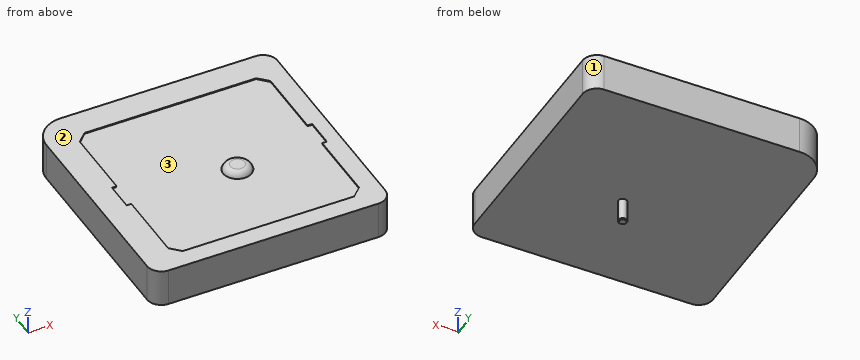
Autodesk Inventor part; units mm, degrees
ref_plane "Work Plane1" through (1.75, -1.75, 0) normal (1, 0, 0) x (0, 1, 0)
ref_plane "XZ Plane" through (0, 0, 0) normal (0, 1, 0) x (-1, 0, 0)
ref_plane "XY Plane" through (0, 0, 0) normal (0, 0, 1) x (1, 0, 0)
sketch "Sketch1" plane through (0, 0, 0) normal (0, 0, 1) x (1, 0, 0)
  line L0 (-11.05, -12.55) -> (11.05, -12.55)
  line L1 (12.55, -11.05) -> (12.55, 11.05)
  line L2 (11.05, 12.55) -> (-9.55, 12.55)
  line L3 (-12.55, 9.55) -> (-12.55, -11.05)
  line L4 (-12.55, -12.55) -> (12.55, 12.55) construction
  line L5 (12.55, -12.55) -> (-12.55, 12.55) construction
  arc A0 (-9.55, 12.55) -> (-12.55, 9.55) centre (-9.55, 9.55) ccw
  arc A1 (-12.55, -11.05) -> (-11.05, -12.55) centre (-11.05, -11.05) ccw
  arc A2 (11.05, -12.55) -> (12.55, -11.05) centre (11.05, -11.05) ccw
  arc A3 (12.55, 11.05) -> (11.05, 12.55) centre (11.05, 11.05) ccw
  circle A4 centre (1.75, -1.75) radius 0.45
  point P0 (0, 0)
  point P1 (0, 0)
  dimension "d0" = 25.1
  dimension "d1" = 3
  dimension "d2" = 0.9
  dimension "d7" = 1.5
  dimension "d8" = 25.1
  dimension "d9" = 1.75
extrude "Extrusion1" add sketch "Sketch1" along normal mid plane 4 contours A1 L3 A0 L2 A3 L1 A2 L0 | A4
extrude "Extrusion2" add sketch "Sketch1" against normal blind 4.4 and the other way blind 2.25 contours A4
chamfer "Chamfer1" distance 0.1 angle 45 1 edges at (1.3, -1.75, -4.4)
sketch "Sketch4" plane through (0, 0, 2) normal (0, 0, 1) x (1, 0, 0)
  line L0 (-12.55, 9.55) -> (-12.55, -11.05)
  arc A0 (-12.55, -11.05) -> (-11.05, -12.55) centre (-11.05, -11.05) ccw
  line L1 (-11.05, -12.55) -> (11.05, -12.55)
  arc A1 (11.05, -12.55) -> (12.55, -11.05) centre (11.05, -11.05) ccw
  line L2 (12.55, -11.05) -> (12.55, 11.05)
  arc A2 (12.55, 11.05) -> (11.05, 12.55) centre (11.05, 11.05) ccw
  line L3 (11.05, 12.55) -> (-9.55, 12.55)
  arc A3 (-9.55, 12.55) -> (-12.55, 9.55) centre (-9.55, 9.55) ccw
  line L4 (-8.55, 9.55) -> (9.55, 9.55)
  line L5 (10.55, 8.55) -> (10.55, -9.55)
  line L6 (9.55, -10.55) -> (-8.55, -10.55)
  line L7 (-9.55, -9.55) -> (-9.55, 8.55)
  line L8 (-8.55, 9.55) -> (-9.55, 8.55)
  line L9 (9.55, 9.55) -> (10.55, 8.55)
  line L10 (10.55, -9.55) -> (9.55, -10.55)
  line L11 (-8.55, -10.55) -> (-9.55, -9.55)
  line L12 (-9.55, 1) -> (-10.05, 1)
  line L13 (-10.05, 1) -> (-10.05, -2)
  line L14 (-10.05, -2) -> (-9.55, -2)
  line L15 (-9.55, -2) -> (-9.55, 1)
  line L16 (10.55, 1) -> (11.05, 1)
  line L17 (11.05, 1) -> (11.05, -2)
  line L18 (11.05, -2) -> (10.55, -2)
  line L19 (10.55, -2) -> (10.55, 1)
  point P0 (0, 0)
  point P1 (10.55, -10.55)
  point P2 (10.55, 9.55)
  point P3 (-9.55, -10.55)
  point P4 (10.55, -0.5)
  point P5 (-9.55, -0.5)
  dimension "d21" = 1
  dimension "d22" = 1
  dimension "d23" = 1
  dimension "d24" = 1
  dimension "d25" = 1
  dimension "d26" = 1
  dimension "d27" = 1
  dimension "d28" = 1
  dimension "d29" = 2
  dimension "d30" = 2
  dimension "d31" = 3
  dimension "d32" = 3
  dimension "d33" = 0.5
  dimension "d34" = 3
extrude "Extrusion3" cut sketch "Sketch4" against normal blind 0.1 contours L4 L9 L5 L10 L6 L11 L7 L8 | L7 L14 L13 L12 | L16 L17 L18 L5
ref_plane "Work Plane1" through (1.75, -1.75, 0) normal (1, 0, 0) x (0, 1, 0)
sketch "Sketch5" plane through (1.75, -1.75, 0) normal (1, 0, 0) x (0, 1, 0)
  line L0 (10.3, 1.9) -> (2.75, 1.9)
  line L1 (11.3, 1.9) -> (10.3, 1.9)
  line L2 (10.3, 1.9) -> (11.3, 1.9)
  line L3 (2.75, 1.9) -> (10.3, 1.9)
  line L4 (-0.25, 1.9) -> (2.75, 1.9)
  line L5 (-7.8, 1.9) -> (-0.25, 1.9)
  line L6 (-8.8, 1.9) -> (-7.8, 1.9)
  line L7 (-7.8, 1.9) -> (-8.8, 1.9)
  line L8 (-0.25, 1.9) -> (-7.8, 1.9)
  line L9 (2.75, 1.9) -> (-0.25, 1.9)
  arc A0 (-0.75, 2.5) -> (-1.5, 1.9) centre (-0.75, 1.7312) ccw
  arc A1 (1.5, 1.9) -> (0.75, 2.5) centre (0.75, 1.7312) ccw
  line L10 (-0.75, 2.5) -> (0.75, 2.5)
  line L11 (0.45, -2) -> (-0.45, -2)
  line L12 (-0.45, -4.3) -> (0.45, -4.3)
  line L13 (0, 2.5) -> (0, 1.9)
  point P0 (1.75, 0)
  point P1 (0, -2)
  dimension "d37" = 1.5
  dimension "d38" = 3
  dimension "d39" = 0.6
revolve "Revolution2" add sketch "Sketch5" angle 360 about axis through (1.75, -1.75, 2.5) along (0, 0, -1) contours L13 L10 A1 L4
sketch "Sketch6" plane through (0, 0, 1.9) normal (0, 0, 1) x (1, 0, 0)
  circle A0 centre (1.75, -1.75) radius 1.5
  line L0 (10.55, 1) -> (11.05, 1)
  line L1 (10.55, 8.55) -> (10.55, 1)
  line L2 (9.55, 9.55) -> (10.55, 8.55)
  line L3 (-8.55, 9.55) -> (9.55, 9.55)
  line L4 (-9.55, 8.55) -> (-8.55, 9.55)
  line L5 (-9.55, 1) -> (-9.55, 8.55)
  line L6 (-10.05, 1) -> (-9.55, 1)
  line L7 (-10.05, -2) -> (-10.05, 1)
  line L8 (-9.55, -2) -> (-10.05, -2)
  line L9 (-9.55, -9.55) -> (-9.55, -2)
  line L10 (-8.55, -10.55) -> (-9.55, -9.55)
  line L11 (9.55, -10.55) -> (-8.55, -10.55)
  line L12 (10.55, -9.55) -> (9.55, -10.55)
  line L13 (10.55, -2) -> (10.55, -9.55)
  line L14 (11.05, -2) -> (10.55, -2)
  line L15 (11.05, 1) -> (11.05, -2)
  circle A1 centre (1.75, -1.75) radius 2
  point P0 (0, 0)
  dimension "d41" = 4
split_face "Split1"
equation "\"d8\" = d0"
equation "\"d30\" = d29"
properties part number "Antenna_GPSPatch" material "Porcelain, Linen"
Work out the finished part from the listing and answer in its coordinate system (mm). Face numbers are marked on the shaded views. Coordinates: 2 decimals unless noted, no trailing zeros. Order: outer loops, then holes, each group sorted by start corner. A loop starts at its lowest first (then second) coordinate and runs counter-clockwise, first axis right, second up. Notation, with made-up numbers: M 3.5,-13 L 52.5,-13 A19 ccw 52.5,6 Z; hole C -38.5,-17.75 d1. An arc over 180 degrees is marked long. Use CSV: the item, a comma, the result in double quotes.
1) Section B-B on x = 10.25 is taken. Write down the section's boundary in (y, z).
Worked out:
outline,"M -12.55,-2 L 12.55,-2 L 12.55,2 L 8.85,2 L 8.85,1.9 L -9.85,1.9 L -9.85,2 L -12.55,2 Z"
2) Determine the mould class of the marked faces 1, 2 and 3 for opening direction X: released by +X, released by -X, zero draft, split by the parting line, or undercut.
Worked out:
face 1,"released by +X"
face 2,"zero draft"
face 3,"undercut"
3) Consider line 1 (Z direction, x = -2.25, y = 6); line 2 (Z direction, x = 2.75, y = -10.75); line 3 (X direction, y = 11.5, z = -0.25). Determine where each line is inside the solid, lowest interval first. Write a range as [from, to].
Worked out:
line 1,"z = [-2, 1.9]"
line 2,"z = [-2, 2]"
line 3,"x = [-11.83, 12.48]"
4) Section C-C on z = -2.5 is taken. Write down the section's boundary in (x, y), plus the area to 3 significant figures.
Worked out:
outline,"C 1.75,-1.75 d0.9"
area,"0.636 mm^2"
5) Section A-A on y = -7.25 is taken. Write down the section's boundary in (x, z), plus the area to 3 significant figures.
Worked out:
outline,"M -12.55,-2 L 12.55,-2 L 12.55,2 L 10.55,2 L 10.55,1.9 L -9.55,1.9 L -9.55,2 L -12.55,2 Z"
area,"98.4 mm^2"
6) Flat-ended cylindrical pins translate along their axes: pin 1 Ø6 at (x, y) = (-3, 3) entering from +Z; pin 2 Ø7.5 at (x, y) = (-2.5, -4.5) entering from +Z. Find the tip coordinate at first contact, or state that the pin passes through.
Worked out:
pin 1,"stops at z = 1.9"
pin 2,"stops at z = 2.26"
